Autodesk Inventor part; units mm, degrees
ref_plane "작업 평면1" through (140, -40, 0) normal (1, 0, 0) x (0, 0, -1)
ref_plane "작업 평면2" through (140, -40, 0) normal (1, 0, 0) x (0, 0, -1)
ref_plane "YZ Plane" through (0, 0, 0) normal (1, 0, 0) x (0, 1, 0)
sketch "스케치1" plane through (0, 0, 0) normal (0, 0, 1) x (1, 0, 0)
  line L0 (0, 10) -> (0, 0)
  line L1 (-10, 10) -> (-10, 20)
  line L2 (-10, 20) -> (290, 20)
  line L3 (290, 20) -> (290, 10)
  line L4 (0, 0) -> (280, 0)
  line L5 (290, 10) -> (290, -40)
  line L6 (-10, 10) -> (-10, -40)
  line L7 (-10, -40) -> (290, -40)
  line L8 (0, 10) -> (10, 10)
  line L9 (10, 10) -> (10, 20)
  line L10 (140, 20) -> (140, 10)
  line L11 (0, 0) -> (-10, 0)
  line L12 (280, 10) -> (280, 0)
  line L13 (280, 10) -> (270, 10)
  line L14 (270, 10) -> (270, 20)
  line L15 (280, 0) -> (290, 0)
  point P0 (140, 0)
  dimension "d2" = 10
  dimension "d5" = 10
  dimension "d6" = 300
  dimension "d9" = 60
  dimension "d12" = 10
  dimension "d13" = 10
extrude "돌출1" add sketch "스케치1" along normal blind 25 contours L8 L9 L2 L14 L13 L12 L4 L0 | L0 L11 L6 L1 L2 L9 L8 | L12 L13 L14 L2 L3 L5 L15
extrude "돌출2" add sketch "스케치1" along normal blind 10 contours L8 L9 L2 L14 L13 L12 L4 L0 | L4 L15 L5 L7 L6 L11
extrude "돌출3" add sketch "스케치1" along normal blind 75 contours L0 L11 L6 L1 L2 L9 L8 | L12 L13 L14 L2 L3 L5 L15
sketch "스케치2" plane through (-10, -40, 0) normal (-1, 0, 0) x (0, 0, 1)
  line L0 (0, 60) -> (0, 0)
  line L1 (0, 0) -> (10, 0)
  line L2 (10, 40) -> (10, 0)
  line L3 (10, 40) -> (75, 40)
  line L4 (75, 60) -> (75, 40)
  line L5 (0, 60) -> (75, 60)
  line L6 (75, 40) -> (10, 0)
  point P0 (0, 40)
extrude "돌출4" add sketch "스케치2" against normal up to surface (10 mm away) contours L2 L3 L6
ref_plane "작업 평면1" through (140, -40, 0) normal (1, 0, 0) x (0, 0, -1)
mirror "미러1" about plane through (140, -40, 0) normal (1, 0, 0) of "돌출4"
sketch "스케치3" plane through (0, 0, 10) normal (0, 0, 1) x (1, 0, 0)
  circle A0 centre (160, -10) radius 2.5
  circle A1 centre (270, -10) radius 2.5
  line L0 (270, 20) -> (10, 20)
  line L1 (290, -40) -> (290, 0)
  line L2 (-10, -40) -> (-10, 0)
  circle A2 centre (160, -30) radius 2.5
  circle A3 centre (270, -30) radius 2.5
  line L3 (140, 20) -> (140, -10)
  point P0 (0, 0)
  dimension "d18" = 30
  dimension "d19" = 5
  dimension "d20" = 20
  dimension "d24" = 5
  dimension "d25" = 20
  dimension "d38" = 20
extrude "돌출5" cut sketch "스케치3" against normal through all
sketch "스케치4" plane through (-10, 20, 0) normal (0, 1, 0) x (1, 0, 0)
  line L0 (280, -25) -> (280, -75)
  line L1 (20, -25) -> (20, -75)
  line L2 (280, -25) -> (20, -25)
  point P0 (10, 0)
  point P1 (35, -20)
  point P2 (265, -20)
  dimension "d26" = 15
  dimension "d27" = 15
  dimension "d28" = 5
hole "구멍1" at (25, 20, 20) at (255, 20, 20) direction (0, -1, 0) diameter 3 end through all counterbore diameter 5 counterbore depth 5
ref_plane "작업 평면2" through (140, -40, 0) normal (1, 0, 0) x (0, 0, -1)
sketch "스케치5" plane through (140, -40, 0) normal (1, 0, 0) x (0, 0, -1)
  line L0 (0, 0) -> (-10, 0)
  line L1 (0, 0) -> (0, 60)
  line L2 (0, 60) -> (-75, 60)
  line L3 (-75, 40) -> (-75, 60)
  line L4 (-10, 0) -> (-75, 40)
  point P0 (0, 40)
extrude "돌출6" cut sketch "스케치5" against normal through all
properties part number "ModuleConnectorRight"
Model file for the job. Use its own axes, mm. A direction names the side the tool comes from. Round coordinates to 2 decimals unless told otherwise and drop trailing zeros. Order: outer loops, then holes, each group sorted by start corner. A loop starts at its lowest first (then second) coordinate and runs counter-clockwise, first axis right, second up.
(1) Drill centre lines: line 1 (Y direction, x = 160, z = 7); line 2 (Z direction, x = 255, y = 16.3); line 3 (Z direction, x = 229, y = 2). Where is each one in solid material? Low to high.
(2) Band-saw the part on B-B (x = 160). List the corners of the cut face in (y, z).
(3) Band-saw the part on D-D (z = 20). List the corners of the cut face in (x, y), then the cut area to 3 significant figures.
(4) 3-axis set-ups, long thin cutter, end or side, ignore diameter. For faces 1 (the face through (255, 15, 22)), 2 (the face through (282, 12, 75)), 3 (the face through (209, -20, 10)): which of +Z, -Z, +X, -X, +Y, -Y reach the whole face in a straight line?
(5) Pull direction X, two halves, no side cores. Call faces 4 (the face through (209, 10, 25)), 5 (the face through (290, -3, 30)), 6 (the face through (272.31, -10.96, 5.07)): released by +X, released by -X, zero draft, split by the parting line, or undercut.
(6) Band-saw the part on C-C (x = 255). List the corners of the cut face in (y, z).
(7) Band-saw the part on A-A (y = -30). List the corners of the cut face in (x, z), then the cut area to 3 significant figures.
(8) Pin check, flat tips, straight feed: pin 1 (10 mm diameter, centred on x = 250, y = -9.5, fed in from -Z); pin 2 (3 mm diameter, centred on x = 160, y = -10, fed in from +Z); pin 3 (6 mm diameter, centred on x = 214.5, y = 7, fed in from +Z); pin 4 (6 mm diameter, centred on x = 270, y = -10, fed in from +Z). Stop position of each tip, or through.
Verdict:
1. line 1: y = -40 to -32.5, -27.5 to -12.5, -7.5 to 20
1. line 2: z = 0 to 17.5, 22.5 to 25
1. line 3: z = 0 to 25
2. outline: (-40, 0) - (-32.5, 0) - (-32.5, 10) - (-40, 10) - close; (-27.5, 0) - (-12.5, 0) - (-12.5, 10) - (-27.5, 10) - close; (-7.5, 0) - (20, 0) - (20, 25) - (0, 25) - (0, 10) - (-7.5, 10) - close
3. outline: (140, 0) - (253.5, 0) - (253.5, 15) - (252.5, 15) - (252.5, 20) - (140, 20) - close; (256.5, 0) - (280, 0) - (280, -33.85) - (290, -33.85) - (290, 20) - (257.5, 20) - (257.5, 15) - (256.5, 15) - close
3. area: 3,270 mm2
4. face 1: +Y
4. face 2: +Z, +X, -X, +Y, -Y
4. face 3: +Z, -X, -Y
5. face 4: zero draft
5. face 5: released by +X
5. face 6: undercut
6. outline: (-40, 0) - (20, 0) - (20, 17.5) - (15, 17.5) - (15, 18.5) - (0, 18.5) - (0, 10) - (-40, 10) - close; (0, 21.5) - (15, 21.5) - (15, 22.5) - (20, 22.5) - (20, 25) - (0, 25) - close
7. outline: (140, 0) - (157.5, 0) - (157.5, 10) - (140, 10) - close; (162.5, 0) - (267.5, 0) - (267.5, 10) - (162.5, 10) - close; (272.5, 0) - (290, 0) - (290, 26.25) - (280, 26.25) - (280, 10) - (272.5, 10) - close
7. area: 1,560 mm2
8. pin 1: stops at z = 0
8. pin 2: passes through
8. pin 3: stops at z = 25
8. pin 4: stops at z = 10
